Could you check a few things on this model? Use its own coordinates, in mm. A direction names the side the tool comes from. Give positions to 0.01 mm unless a question says otherwise; leave off trailing zeros. Loops run counter-clockwise (first coordinate to the right, second up) from the corner with the lowest first, then second, coordinate; pieces in that order, holes last. Notation, with made-up numbers: (63.25, 17.5) -> (73.25, 17.5) arc R17 cw to (73.25, 42.5) -> close; hole circle Ø1 at (-36, 25.5). An arc over 180 degrees is marked (long way). Write each question's results on one line, items separated by ' | '. Start each with the question number.
Q1. Which directions (+Z, -Z, +X, -X, +Y, -Y) give clear straight access to the entire face, cutting with the end or side of a thin tool? Please do faces 1 (the face through (-28, 4, 0)), 2 (the face through (17, 4, 24)), 3 (the face through (-32, -3.8, -0.1)), 4 (the face through (33, 6, -10)).
Q2. If we section it at C-C, the plane y = -5: List the corners of the cut face in (x, z) for me, plus the area to 3 significant figures.
Q3. If we section it at D-D, the plane z = -24: List the corners of the cut face in (x, y) for me, plus the area to 3 significant figures.
Q4. Will these pins go through, and if not, where does the flat tip stop? P1, Ø4, axis at y = 4, z = -26, coming from the +X side; P2, Ø1.5, axis at x = 22, y = 6, coming from the +Z side; P3, Ø1, axis at y = -0.5, z = -5, coming from the -X side.
Q5. If we section it at A-A, the plane y = 5.5: List the corners of the cut face in (x, z) for me.
Q6. If we section it at B-B, the plane x = 0: List the corners of the cut face in (y, z) for me.
Q7. If I drill on line 1 along Y through (x, z) = (-30.05, 0); line 2 along X through (y, z) = (5, -7.5); line 3 along Z through (x, y) = (33.75, -5), over which ranges is the centre line in solid material (lowest first)?
Q8. We'd pull the mould along Z, two halves only. Please class faces 5 (the face through (-33, -5, -10)), 6 (the face through (0, 1, 18.75)), 7 (the face through (-18, 8, -21)): released by +Z, released by -Z, zero draft, split by the parting line, or undercut.
Autodesk Inventor part; units mm, degrees
ref_plane "YZ Plane" through (0, 0, 0) normal (1, 0, 0) x (0, 1, 0)
ref_plane "XZ Plane" through (0, 0, 0) normal (0, 1, 0) x (-1, 0, 0)
ref_plane "XY Plane" through (0, 0, 0) normal (0, 0, 1) x (1, 0, 0)
sketch "Szkic1" plane through (0, 0, 0) normal (0, 1, 0) x (-1, 0, 0)
  circle A0 centre (0, 0) radius 35.5
  line L0 (0, 18.75) -> (0, -18.75) construction
  line L1 (-28, 0) -> (28, 0) construction
  line L2 (-28, -18.75) -> (28, -18.75)
  line L3 (-28, 18.75) -> (-28, -18.75)
  line L4 (28, 18.75) -> (28, -18.75)
  line L5 (0, 18.75) -> (28, 18.75)
  line L6 (0, 18.75) -> (-28, 18.75)
  line L7 (0, 18.75) -> (0, 28.75) construction
  line L8 (17, 28.75) -> (-17, 28.75)
  line L9 (17, 28.75) -> (17, 18.75)
  line L10 (-17, 28.75) -> (-17, 18.75)
  line L11 (0, -18.75) -> (0, -28.75) construction
  line L12 (-17, -28.75) -> (17, -28.75)
  line L13 (17, -28.75) -> (17, -18.75)
  line L14 (-17, -28.75) -> (-17, -18.75)
  dimension "d0" = 71
  dimension "d1" = 37.5
  dimension "d2" = 56
  dimension "d3" = 10
  dimension "d4" = 34
  dimension "d5" = 10
  dimension "d6" = 34
extrude "Wyciągnięcie proste1" add sketch "Szkic1" along normal blind 2 contours L3 L6 L5 L4 L2
extrude "Wyciągnięcie proste2" add sketch "Szkic1" along normal blind 8
sketch "Szkic2" plane through (0, 0, 0) normal (0, -1, 0) x (1, 0, 0)
  line L0 (32, 0) -> (-32, 0) construction
  circle A0 centre (0, 0) radius 35.5
  line L1 (-32, -10) -> (-32, 10)
  line L2 (32, -10) -> (32, 10)
  line L3 (32, -10) -> (34.0624, -10)
  line L4 (32, 10) -> (34.0624, 10)
  line L5 (-32, -10) -> (-34.0624, -10)
  line L6 (-32, 10) -> (-34.0624, 10)
  dimension "d11" = 64
  dimension "d12" = 71
  dimension "d13" = 20
  dimension "d14" = 20
extrude "Wyciągnięcie proste3" add sketch "Szkic2" along normal blind 10 contours A0 L3 L2 L4 | L6 L1 L5 A0
sketch "Szkic3" plane through (32, 0, -10) normal (-1, 0, 0) x (0, 0, 1)
  line L0 (10, 0) -> (10, -5) construction
  circle A0 centre (10, -5) radius 1
  dimension "d17" = 5
  dimension "d18" = 2
extrude "Wyciągnięcie proste4" cut sketch "Szkic3" along normal through all both and the other way through all
sketch "Szkic4" plane through (0, 2, 0) normal (0, 1, 0) x (1, 0, 0)
  line L0 (-10.2735, 0) -> (10.2735, 0) construction
  line L1 (0, 9.2596) -> (0, -9.2596) construction
  point P0 (0, 0)
sketch "Szkic5" plane through (0, 8, 0) normal (0, 1, 0) x (1, 0, 0)
  line L0 (32, 0) -> (-32, 0) construction
  circle A0 centre (0, 0) radius 35.5
  line L1 (-32, -10) -> (-32, 10)
  line L2 (32, -10) -> (32, 10)
  line L3 (32, -10) -> (34.0624, -10)
  line L4 (32, 10) -> (34.0624, 10)
  line L5 (-32, -10) -> (-34.0624, -10)
  line L6 (-32, 10) -> (-34.0624, 10)
  dimension "d21" = 64
  dimension "d22" = 71
  dimension "d23" = 20
  dimension "d24" = 20
extrude "Wyciągnięcie proste5" cut sketch "Szkic5" against normal blind 5 contours A0 L3 L2 L4 | L6 L1 L5 A0
sketch "Szkic6" plane through (32, 8, 10) normal (1, 0, 0) x (0, 0, -1)
  line L0 (10, -8) -> (10, -2.5) construction
  circle A0 centre (10, -2.5) radius 1
  dimension "d27" = 5.5
  dimension "d28" = 2
extrude "Wyciągnięcie proste6" cut sketch "Szkic6" against normal through all
properties part number "003-001"
Final values:
1) face 1: +Y | face 2: +Y, -Y | face 3: +Z, -Z, -Y | face 4: +X, +Y
2) outline: (-35.49, -1) arc R35.5 ccw to (-34.06, -10) -> (-32, -10) -> (-32, -1) -> close; (-35.49, 1) -> (-32, 1) -> (-32, 10) -> (-34.06, 10) arc R35.5 ccw to start; (32, -10) -> (34.06, -10) arc R35.5 ccw to (35.49, -1) -> (32, -1) -> close; (32, 1) -> (35.49, 1) arc R35.5 ccw to (34.06, 10) -> (32, 10) -> close | area: 107 mm²
3) outline: (-26.16, 0) -> (-17, 0) -> (-17, 8) -> (-26.16, 8) -> close; (17, 0) -> (26.16, 0) -> (26.16, 8) -> (17, 8) -> close | area: 147 mm²
4) P1: stops at x = 26.16 | P2: stops at z = 28.44 | P3: stops at x = -35.21
5) outline: (-34.06, -10) arc R35.5 ccw to (34.06, -10) -> (32, -10) -> (32, -1) -> (28, -1) -> (28, -18.75) -> (17, -18.75) -> (17, -28.75) -> (-17, -28.75) -> (-17, -18.75) -> (-28, -18.75) -> (-28, -1) -> (-32, -1) -> (-32, -10) -> close; (-34.06, 10) -> (-32, 10) -> (-32, 1) -> (-28, 1) -> (-28, 18.75) -> (-17, 18.75) -> (-17, 28.75) -> (17, 28.75) -> (17, 18.75) -> (28, 18.75) -> (28, 1) -> (32, 1) -> (32, 10) -> (34.06, 10) arc R35.5 ccw to start
6) outline: (0, -35.5) -> (8, -35.5) -> (8, -28.75) -> (0, -28.75) -> close; (0, -18.75) -> (2, -18.75) -> (2, 18.75) -> (0, 18.75) -> close; (0, 28.75) -> (8, 28.75) -> (8, 35.5) -> (0, 35.5) -> close
7) line 1: y = 0 to 4.5, 6.5 to 8 | line 2: x = -32 to -28, 28 to 32 | line 3: z = -10 to -1, 1 to 10
8) face 5: released by -Z | face 6: undercut | face 7: zero draft
